```python
from build123d import *

# Parameters (mm, degrees)
SKETCH_1_R          = 1.6
SKETCH_1_W          = 50.5
SKETCH_1_H          = 53.910884284
EXTRUDE_1_DEPTH     = 3
CUT_EXTRUDE_1_DEPTH = 4


with BuildPart() as part:
    # ｽｹｯﾁ1 → ﾎﾞｽ - 押し出し1 (new body)
    with BuildSketch(Plane.XY):
        Polygon((-36.39879245, 96.955442142), (36.39879245, 96.955442142), (102.165272155, -16.955442142), (65.766479705, -80), (-65.766479705, -80), (-102.165272155, -16.955442142), align=None)
        with Locations((30.25, 91.195498156)):
            Circle(SKETCH_1_R, mode=Mode.SUBTRACT)
        with Locations((30.25, 41.195498156)):
            Circle(SKETCH_1_R, mode=Mode.SUBTRACT)
        with Locations((-30.25, 41.195498156)):
            Circle(SKETCH_1_R, mode=Mode.SUBTRACT)
        with Locations((-30.25, 91.195498156)):
            Circle(SKETCH_1_R, mode=Mode.SUBTRACT)
        with Locations((63.852618114, -71.795017542)):
            Circle(SKETCH_1_R, mode=Mode.SUBTRACT)
        with Locations((94.102618114, -19.400480613)):
            Circle(SKETCH_1_R, mode=Mode.SUBTRACT)
        with Locations((50.801347925, 5.599519387)):
            Circle(SKETCH_1_R, mode=Mode.SUBTRACT)
        with Locations((20.551347925, -46.795017542)):
            Circle(SKETCH_1_R, mode=Mode.SUBTRACT)
        with Locations((-94.102618114, -19.400480613)):
            Circle(SKETCH_1_R, mode=Mode.SUBTRACT)
        with Locations((-63.852618114, -71.795017542)):
            Circle(SKETCH_1_R, mode=Mode.SUBTRACT)
        with Locations((-20.551347925, -46.795017542)):
            Circle(SKETCH_1_R, mode=Mode.SUBTRACT)
        with Locations((-50.801347925, 5.599519387)):
            Circle(SKETCH_1_R, mode=Mode.SUBTRACT)
        with Locations((-45, 57)):
            Circle(SKETCH_1_R, mode=Mode.SUBTRACT)
        with Locations((45, 57)):
            Circle(SKETCH_1_R, mode=Mode.SUBTRACT)
        with Locations((45, -73)):
            Circle(SKETCH_1_R, mode=Mode.SUBTRACT)
        with Locations((-45, -73)):
            Circle(SKETCH_1_R, mode=Mode.SUBTRACT)
        Circle(SKETCH_1_R, mode=Mode.SUBTRACT)
        with Locations((0, 60)):
            Rectangle(SKETCH_1_W, SKETCH_1_H, mode=Mode.SUBTRACT)
        Polygon((87.930621892, -21.610579625), (62.680621892, -65.344862517), (15.992426562, -38.389420375), (41.242426562, 5.344862517), align=None, mode=Mode.SUBTRACT)
        Polygon((-62.680621892, -65.344862517), (-87.930621892, -21.610579625), (-41.242426562, 5.344862517), (-15.992426562, -38.389420375), align=None, mode=Mode.SUBTRACT)
    extrude(amount=EXTRUDE_1_DEPTH)

    # ｽｹｯﾁ2 → ｶｯﾄ - 押し出し1 (cut, through all)
    with BuildSketch(Plane.XY.offset(3)):
        with BuildLine():
            Line((-10.828203914, 33.044557858), (10.828203914, 33.044557858))
            ThreePointArc((10.828203914, 33.044557858), (0, 29.544557858), (-10.828203914, 33.044557858))
        make_face()
        with BuildLine():
            Line((34.031528519, -7.144779262), (23.203324605, -25.899778596))
            ThreePointArc((23.203324605, -25.899778596), (25.586337649, -14.772278929), (34.031528519, -7.144779262))
        make_face()
        with BuildLine():
            Line((-23.203324605, -25.899778596), (-34.031528519, -7.144779262))
            ThreePointArc((-34.031528519, -7.144779262), (-25.586337649, -14.772278929), (-23.203324605, -25.899778596))
        make_face()
    extrude(amount=-CUT_EXTRUDE_1_DEPTH, mode=Mode.SUBTRACT)


solid = part.part
```
Source: CAD feature listing. Evaluate the final solid. Frame: model axes, mm. A direction names the side the tool comes from. Give positions to 0.01 mm unless a question says otherwise; leave off trailing zeros. Order: outer loops, then holes, each group sorted by start corner. A loop starts at its lowest first (then second) coordinate and runs counter-clockwise, first axis right, second up. Notation, with made-up numbers: (67, 39) -> (94, 39) arc R19 cw to (94, 48) -> close; hole circle Ø5 at (52, -9). An arc over 180 degrees is marked (long way). Use a Markdown table: item, result.
Q1. Material intervals for line 1 (Y direction, x = 0, z = 1.85); line 2 (X direction, y = -41.5, z = 2.3); line 3 (X direction, y = 56, z = 2.1), sorted ascending. Write a range as [from, to].
A:
| item | result |
|---|---|
| line 1 | [-80, -1.6], [1.6, 29.54], [86.96, 96.96] |
| line 2 | [-87.99, -76.45], [-21.38, 21.38], [76.45, 87.99] |
| line 3 | [-60.04, -46.25], [-43.75, -25.25], [25.25, 43.75], [46.25, 60.04] |
Q2. First-contact query: P1, Ø5, axis at x = -63.85, y = -71.8, coming from the +Z side; P2, Ø1.5, axis at y = 60.5, z = 1, coming from the +X side; P3, Ø1, axis at x = -51, z = 1.5, coming from the +Y side; P4, Ø1, axis at y = 39, z = 2.5, coming from the -X side. Flat tips, straight axial feed; report the tip coordinate or a pass-through.
A:
| item | result |
|---|---|
| P1 | z = 3 |
| P2 | x = 57.88 |
| P3 | y = 72.53 |
| P4 | x = -70.15 |
Q3. Pull-direction query (Y, two-part tool) for faces 3 (the face through (1, -10, 3)), 4 (the face through (39.663, -52.056, 1.479)), 5 (the face through (-83.71, -48.92, 1.48)); classes: +Y half, -Y half, draft (parallel to the pull), parting line (faces both ways), or undercut.
A:
| item | result |
|---|---|
| face 3 | draft |
| face 4 | undercut |
| face 5 | -Y half |
Q4. Access query for faces 1 (the face through (-37.69, -0.81, 1.48)), 2 (the face through (68.82, 40.8, 1.48)). Directions: +Z, -Z, +X, -X, +Y, -Y. A direction counts if a zero-diameter tool reaches every point of the face in a straight line with its end or side. Return the directions, or none.
A:
| item | result |
|---|---|
| face 1 | +Z, -Z |
| face 2 | +Z, -Z, +X, +Y |
Q5. Section B-B (y = 64). Return the cut outline in (x, z).
A:
| item | result |
|---|---|
| outline | (-55.43, 0) -> (-25.25, 0) -> (-25.25, 3) -> (-55.43, 3) -> close; (25.25, 0) -> (55.43, 0) -> (55.43, 3) -> (25.25, 3) -> close |
Q6. Section A-A (y = -35). Return the cut outline in (x, z).
A:
| item | result |
|---|---|
| outline | (-91.75, 0) -> (-80.2, 0) -> (-80.2, 3) -> (-91.75, 3) -> close; (-17.95, 0) -> (17.95, 0) -> (17.95, 3) -> (-17.95, 3) -> close; (80.2, 0) -> (91.75, 0) -> (91.75, 3) -> (80.2, 3) -> close |
Q7. Section C-C (z = 1.45). State how many separate pieces and enclosed holes the cut face has, and give its area (3 significant figures).
A:
| item | result |
|---|---|
| separate pieces | 1 |
| enclosed holes | 20 |
| area | 17,900 mm^2 |
